from build123d import *

# Parameters (mm, degrees)
FLANGE_BASE1_DEPTH    = 12.5
ESBO_O3_R             = 5
CORTE_EXTRUS_O1_DEPTH = 10


# Sheet-metal steps are written as plain solids
with BuildPart() as part:
    # Esboço1 → Flange-base1 (new, symmetric)
    with BuildSketch(Plane.XY):
        with BuildLine():
            Line((0, 0), (0, -19.229670386))
            ThreePointArc((0, -19.229670386), (0.072174453, -19.98610047), (0.286093236, -20.715233091))
            Line((0.286093236, -20.715233091), (3.856953382, -29.642383454))
            ThreePointArc((3.856953382, -29.642383454), (3.963912773, -30.006949765), (4, -30.385164807))
            Line((4, -30.385164807), (4, -50))
            Line((4, -50), (6, -50))
            Line((6, -50), (6, -30.385164807))
            ThreePointArc((6, -30.385164807), (5.927825547, -29.628734723), (5.713906764, -28.899602102))
            Line((5.713906764, -28.899602102), (2.143046618, -19.972451738))
            ThreePointArc((2.143046618, -19.972451738), (2.036087227, -19.607885428), (2, -19.229670386))
            Line((2, -19.229670386), (2, 0))
            Line((2, 0), (0, 0))
        make_face()
    extrude(amount=FLANGE_BASE1_DEPTH, both=True)

    # Esboço3 → Corte-extrusão1 (cut)
    with BuildSketch(Plane(origin=(6, 0, 0), x_dir=(0, 0, -1), z_dir=(1, 0, 0))):
        with Locations(Location((0, -40.192582404, 0), (0, 0, 90))):
            Circle(ESBO_O3_R)
        with Locations(Location((0, -9.614835193, 0), (0, 0, 90))):
            Circle(ESBO_O3_R)
    extrude(amount=-CORTE_EXTRUS_O1_DEPTH, mode=Mode.SUBTRACT)


solid = part.part
Can you work these out from the model? Positions are in its coordinate system, mm. A direction names the side the tool comes from. Coordinates: 2 decimals unless noted, no trailing zeros. Order: outer loops, then holes, each group sorted by start corner. A loop starts at its lowest first (then second) coordinate and runs counter-clockwise, first axis right, second up. Notation, with made-up numbers: M -8.5,-23.5 L 30.5,-23.5 A20 cw 30.5,3.5 Z; hole C 12.25,8 d6. An arc over 180 degrees is marked long. Answer as CSV lines item,"result".
(1) I'm going to push flat-ended pins straight in: pin 1 (4 mm diameter, centred on y = -31, z = 10, fed in from -X); pin 2 (6 mm diameter, centred on y = -27, z = 5.5, fed in from +X); pin 3 (1.5 mm diameter, centred on y = -24, z = 8, fed in from +X). Where does each tip first touch, or does it pass through?
Geometry check:
pin 1,"x = 3.6"
pin 2,"x = 5.98"
pin 3,"x = 4.05"
(2) Suppose I cut it at D-D on x = 1.5. Please give me the cut outline in (y, z).
Geometry check:
outline,"M -23.75,-12.5 L 0,-12.5 L 0,12.5 L -23.75,12.5 Z; hole C -9.61,0 d10"
(3) Please list where these lines run through material, in increasing order: L1, parallel to X at y = -2.5, z = -10.25; L2, parallel to X at y = -35.5, z = -8.75; L3, parallel to Z at x = 0.9, y = -14.
Geometry check:
L1,"0 to 2"
L2,"4 to 6"
L3,"-12.5 to -2.4, 2.4 to 12.5"
(4) Suppose I cut it at B-B on y = -9. Please give me the cut outline in (x, z).
Geometry check:
outline,"M 0,-12.5 L 2,-12.5 L 2,-4.96 L 0,-4.96 Z; M 0,4.96 L 2,4.96 L 2,12.5 L 0,12.5 Z"
(5) Suppose I cut it at A-A on z = 0. Please give me the cut outline in (x, y), plus the area to 3 significant figures.
Geometry check:
outline,"M 0,-19.23 A4 ccw 0.29,-20.72 L 3.86,-29.64 A2 cw 4,-30.39 L 4,-35.19 L 6,-35.19 L 6,-30.39 A4 ccw 5.71,-28.9 L 2.14,-19.97 A2 cw 2,-19.23 L 2,-14.61 L 0,-14.61 Z; M 0,-4.61 L 2,-4.61 L 2,0 L 0,0 Z; M 4,-50 L 6,-50 L 6,-45.19 L 4,-45.19 Z"
area,"61.5 mm^2"
(6) If we mould it in two halves opening along Y, with no side actions, what happens to faces 1 (the cylindrical face through (5.93, -29.64, 0.18)), 2 (the cylindrical face through (5.014, -45.188, 0.22)), 3 (the flat face through (6, -45, 3))? For each: released by +Y, released by -Y, zero draft, split by the parting line, or undercut.
Geometry check:
face 1,"released by +Y"
face 2,"undercut"
face 3,"zero draft"
(7) Suppose I cut it at C-C on z = 5.5. Please give me the cut outline in (x, y), plus the area to 3 significant figures.
Geometry check:
outline,"M 0,-19.23 A4 ccw 0.29,-20.72 L 3.86,-29.64 A2 cw 4,-30.39 L 4,-50 L 6,-50 L 6,-30.39 A4 ccw 5.71,-28.9 L 2.14,-19.97 A2 cw 2,-19.23 L 2,0 L 0,0 Z"
area,"101 mm^2"
(8) On a 3-axis mill with a long thin cutter (end or side, diameter ignored), from which of +Z, -Z, +X, -X, +Y, -Y can I reach the whole of each face in a straight line? I mean faces 4 (the flat face through (1, 0, 0)), 5 (the flat face through (4, -36, 3)), 6 (the flat face through (2, -14, 3)). Say none if no direction works.
Geometry check:
face 4,"+Z, -Z, +X, -X, +Y"
face 5,"+Z, -Z, -X, -Y"
face 6,"+Z, -Z, +X, +Y"
